Check sheet for the modelled part. Datum: model origin and axes. Units: mm. A direction names the side the tool comes from. Coordinates: 2 decimals unless noted, no trailing zeros. Loops run counter-clockwise (first coordinate to the right, second up) from the corner with the lowest first, then second, coordinate; pieces in that order, holes last. Notation, with made-up numbers: (-17, 1.5) -> (35, 1.5) arc R25 cw to (35, 34.5) -> close; hole circle Ø9 at (75, -13.75). An arc over 180 degrees is marked (long way). Use one line per item in the form item = value.
from build123d import *

# Parameters (mm, degrees)
SKETCH008_R     = 6
PAD002_DEPTH    = 24
POCKET_DEPTH    = 20
CHAMFER001_SIZE = 2


with BuildPart() as part:
    # Sketch008 → Pad002 (new body)
    with BuildSketch(Plane.XY.offset(18)):
        Circle(SKETCH008_R)
    extrude(amount=PAD002_DEPTH)

    # Sketch007 (on Face3 of Pad002) → Pocket (cut)
    with BuildSketch(Plane.XY.offset(42)):
        Polygon((5.195447, -3.001222), (0.001411, 6), (-5.196858, -2.998778), align=None)
    extrude(amount=-POCKET_DEPTH, mode=Mode.SUBTRACT)

    # Chamfer001
    chamfer001_edges = [part.edges().sort_by_distance(p)[0] for p in [
        (-6, 0, 18),
    ]]
    chamfer(chamfer001_edges, length=CHAMFER001_SIZE)


solid = part.part
(1) Go/stop test with flat-tipped pins: P1, Ø1.5, axis at x = -2, z = 28.5, coming from the -Y side; P2, Ø2.5, axis at x = 1.5, y = -0.5, coming from the +Z side. Record where each tip stops, or that it passes through.
Established:
P1 = -5.87
P2 = 22
(2) Tool access check on faces 1 (the flat face through (-2.561, 1.564, 32.14)), 2 (the flat face through (-4, 3, 42)). Record the directions out of +Z, -Z, +X, -X, +Y, -Y that give a thin tool (end or side, any length) a straight path to the whole face; none if there is none.
Established:
face_1 = +Z
face_2 = +Z, +X, -X, +Y, -Y
(3) Section check B-B, the plane z = 19.5. Record the boundary of the cut face in (x, y), plus the area to 3 significant figures.
Established:
outline = circle Ø11 at (0, 0)
area = 95.0 mm²
(4) Mould release check, pull along X, two halves, no side actions. Record for faces 3 (the flat face through (0, 0, 18)), 4 (the flat face through (0, 1, 22)), 5 (the cylindrical face through (-6, 0, 31)): +X half, -X half, draft (parallel to the pull), parting line (faces both ways), or undercut.
Established:
face_3 = draft
face_4 = undercut
face_5 = parting line
(5) Scan lines: line 1 along X through (y, z) = (3.25, 28.75); line 2 along Y through (x, z) = (2, 39.5); line 3 along X through (y, z) = (-0.25, 21.25). Record each from-to range of solid material in increasing order.
Established:
line_1 = -5.04 to -1.59, 1.59 to 5.04
line_2 = -5.66 to -3, 2.54 to 5.66
line_3 = -5.99 to 5.99
